from build123d import *

# Parameters (mm, degrees)
SKETCH11_R          = 1.6
CUT_EXTRUDE11_DEPTH = 8
CHAMFER5_SIZE       = 0.2
SKETCH13_R          = 1.75
CUT_EXTRUDE13_DEPTH = 8
CHAMFER4_SIZE       = 0.4


with BuildPart() as part:
    # Sketch1 → Base-Revolve (revolve)
    with BuildSketch(Plane.XY, mode=Mode.PRIVATE) as base_revolve_sk:
        with BuildLine():
            Line((22, 24), (22, 25))
            Line((22, 25), (25, 25))
            Line((25, 25), (25, 7))
            Line((25, 7), (29, 7))
            Line((29, 7), (29, 4))
            Line((29, 4), (25, 4))
            Line((25, 4), (25, 0))
            Line((25, 0), (15, 0))
            Line((15, 0), (15, 0.1))
            Line((15, 0.1), (14.873999475, 0))
            Line((14.873999475, 0), (12.721791982, 0))
            Line((12.721791982, 0), (12.574111279, 0.1))
            Line((12.574111279, 0.1), (12.45924851, 0.1))
            Line((12.45924851, 0.1), (12.357749883, 0))
            Line((12.357749883, 0), (11.190176325, 0))
            Line((11.190176325, 0), (7.701985053, 0))
            Line((7.701985053, 0), (7.511808728, 0.121233853))
            Line((7.511808728, 0.121233853), (7.364301677, 0.121233853))
            Line((7.364301677, 0.121233853), (7.243067824, 0))
            Line((7.243067824, 0), (5.1, 0))
            Line((5.1, 0), (5, 0.1))
            Line((5, 0.1), (5, 0))
            Line((5, 0), (5, -15))
            Line((5, -15), (0, -15))
            Line((0, -15), (0, 24))
            Line((0, 24), (1.934523123, 24))
            Line((1.934523123, 24), (2, 23.918490551))
            Line((2, 23.918490551), (2.075283648, 24))
            Line((2.075283648, 24), (4, 24))
            Line((4, 24), (4, 20))
            Line((4, 20), (6, 20))
            Line((6, 20), (6, 24))
            Line((6, 24), (10, 24))
            ThreePointArc((10, 24), (10.5, 24.207106781), (11, 24))
            Line((11, 24), (22, 24))
        make_face()
    revolve(base_revolve_sk.sketch.rotate(Axis((0, 0, 0), (0, 1, 0)), 90), axis=Axis((0, 0, 0), (0, 1, 0)))

    # Sketch11 → Cut-Extrude11 (cut)
    with BuildSketch(Plane.XZ):
        with Locations(Location((-21, 0, 0), (0, 0, 270))):
            Circle(SKETCH11_R)
        with Locations(Location((10.5, 18.186533479, 0), (0, 0, 270))):
            Circle(SKETCH11_R)
        with Locations(Location((10.5, -18.186533479, 0), (0, 0, 270))):
            Circle(SKETCH11_R)
    extrude(amount=-CUT_EXTRUDE11_DEPTH, mode=Mode.SUBTRACT)

    # Cut-Extrude12 cone 1 section (through the dimple's axis) → Cut-Extrude12 (revolve, cut)
    with BuildSketch(Plane(origin=(10.5, 8, -18.186533479), x_dir=(0, 0, -1), z_dir=(1, 0, 0))):
        Polygon((0, 0), (1.6, 0), (0, 0.923760431), align=None)
    revolve(axis=Axis((10.5, 8, -18.186533479), (0, 1, 0)), mode=Mode.SUBTRACT)

    # Cut-Extrude12 cone 2 section (through the dimple's axis) → Cut-Extrude12 cone 2 (revolve, cut)
    with BuildSketch(Plane(origin=(-21, 8, 0), x_dir=(0, 0, -1), z_dir=(1, 0, 0))):
        Polygon((0, 0), (1.6, 0), (0, 0.923760431), align=None)
    revolve(axis=Axis((-21, 8, 0), (0, 1, 0)), mode=Mode.SUBTRACT)

    # Cut-Extrude12 cone 3 section (through the dimple's axis) → Cut-Extrude12 cone 3 (revolve, cut)
    with BuildSketch(Plane(origin=(10.5, 8, 18.186533479), x_dir=(0, 0, -1), z_dir=(1, 0, 0))):
        Polygon((0, 0), (1.6, 0), (0, 0.923760431), align=None)
    revolve(axis=Axis((10.5, 8, 18.186533479), (0, 1, 0)), mode=Mode.SUBTRACT)

    # Chamfer5
    chamfer5_edges = [part.edges().sort_by_distance(p)[0] for p in [
        (0, 25, 25),
        (0, 25, 22),
        (0, 24, 6),
        (0, 24, 4),
        (0, 0, 25),
        (0, 4, 25),
        (0, 4, 29),
        (0, 7, 29),
        (0, 7, 25),
    ]]
    chamfer(chamfer5_edges, length=CHAMFER5_SIZE)

    # Sketch13 → Cut-Extrude13 (cut)
    with BuildSketch(Plane(origin=(0, 24, 0), x_dir=(-1, 0, 0), z_dir=(0, 1, 0))):
        with Locations(Location((0, -18, 0), (0, 0, 90))):
            Circle(SKETCH13_R)
        with Locations(Location((0, 18, 0), (0, 0, 90))):
            Circle(SKETCH13_R)
    extrude(amount=-CUT_EXTRUDE13_DEPTH, mode=Mode.SUBTRACT)

    # Cut-Extrude14 cone 1 section (through the dimple's axis) → Cut-Extrude14 (revolve, cut)
    with BuildSketch(Plane(origin=(0, 16, -18), x_dir=(0, 0, 1), z_dir=(1, 0, 0))):
        Polygon((0, 0), (1.75, 0), (0, 1.225363192), align=None)
    revolve(axis=Axis((0, 16, -18), (0, -1, 0)), mode=Mode.SUBTRACT)

    # Cut-Extrude14 cone 2 section (through the dimple's axis) → Cut-Extrude14 cone 2 (revolve, cut)
    with BuildSketch(Plane(origin=(0, 16, 18), x_dir=(0, 0, 1), z_dir=(1, 0, 0))):
        Polygon((0, 0), (1.75, 0), (0, 1.225363192), align=None)
    revolve(axis=Axis((0, 16, 18), (0, -1, 0)), mode=Mode.SUBTRACT)

    # Chamfer4
    chamfer4_edges = [part.edges().sort_by_distance(p)[0] for p in [
        (0, 24, -19.75),
        (0, 24, 16.25),
        (0, -15, 5),
        (-21, 0, 1.6),
        (10.5, 0, 19.786533479),
        (10.5, 0, -16.586533479),
    ]]
    chamfer(chamfer4_edges, length=CHAMFER4_SIZE)


solid = part.part
Can you work these out from the model? Positions are in its coordinate system, mm. A direction names the side the tool comes from. Give positions to 0.01 mm unless a question says otherwise; leave off trailing zeros. Loops run counter-clockwise (first coordinate to the right, second up) from the corner with the lowest first, then second, coordinate; pieces in that order, holes last. Notation, with made-up numbers: (32.5, 48) -> (44.5, 48) arc R22 cw to (44.5, 69) -> close; hole circle Ø3 at (26.5, 26). An arc over 180 degrees is marked (long way). Return JSON: item names as keys, results as strings.
Q1. I want a section at A-A, the plane y = 17. List the corners of the cut face in (x, z) for me, then the cut area to 3 significant figures.
Checks:
{"outline": "circle Ø50 at (0, 0); hole circle Ø3.5 at (0, -18); hole circle Ø3.5 at (0, 18)", "area": "1,940 mm2"}
Q2. We'd pull the mould along Z, two halves only. Please class faces 4 (the face through (-10, 24, 5)), 5 (the face through (25.5, 4, 0.1)): released by +Z, released by -Z, zero draft, split by the parting line, or undercut.
Checks:
{"face 4": "undercut", "face 5": "zero draft"}
Q3. For pin 1 Ø3.5 at (x, z) = (-3, -1.5) entering from +Y; pin 2 Ø8 at (x, z) = (18, -19) entering from +Y; pin 3 Ø8 at (y, z) = (5, 12.5) entering from +X; pin 4 Ø1.9 at (x, z) = (-21, 0) entering from -Y, each with a flat end and sliding along its axis, tell me the tip position at first contact or that it passes through.
Checks:
{"pin 1": "stops at y = 24", "pin 2": "stops at y = 25", "pin 3": "stops at x = 27.73", "pin 4": "stops at y = 8.38"}
Q4. On a 3-axis mill with a long thin cutter (end or side, diameter ignored), from which of +Z, -Z, +X, -X, +Y, -Y can I reach the whole of each face in a straight line? I mean faces 1 (the face through (4, 24, -5)), 2 (the face through (0, -15, 0)), 3 (the face through (0, -7, 5)). Say none if no direction works.
Checks:
{"face 1": "+Y", "face 2": "+Z, -Z, +X, -X, -Y", "face 3": "-Y"}
Q5. I need wall thicknesses on probe 1 along X at (y, z) = (21.45, 0); probe 2 along X at (y, z) = (7.5, -20); probe 3 along Y at (x, z) = (-21.5, 2.5). Which ranges of each line are inside material? Lowest first, please.
Checks:
{"probe 1": "x = -25 to -6, -4 to 4, 6 to 25", "probe 2": "x = -15 to 15", "probe 3": "y = 0 to 24"}
